Autodesk Inventor part; units mm, degrees
ref_plane "Work Plane1" through (227.2466, 0, 0) normal (0, 1, 0) x (-1, 0, 0)
ref_plane "YZ Plane" through (0, 0, 0) normal (1, 0, 0) x (0, 1, 0)
ref_plane "XZ Plane" through (0, 0, 0) normal (0, 1, 0) x (-1, 0, 0)
sketch "Sketch1" plane through (0, 0, 0) normal (0, 0, 1) x (1, 0, 0)
  line L0 (0, 0) -> (21, 0)
  line L1 (0, 0) -> (0, 80)
  line L2 (0, 80) -> (21, 80)
  line L3 (21, 80) -> (21, 0)
  line L4 (0, 96) -> (0, -16)
  line L5 (-4.2, 0) -> (25.2, 0)
  dimension "d1" = 160
  dimension "d2" = 21
revolve "Body" add sketch "Sketch1" angle 360 about axis through (0, 0, 0) along (1, 0, 0)
sketch "Sketch2" plane through (0, 0, 0) normal (-1, 0, 0) x (0, 0, 1)
  circle A0 centre (0, 0) radius 80
  point P0 (0, 0)
hole "Thread" at (0, 0, 0) direction (1, 0, 0) diameter 122.8349 end through all
chamfer "Chamfer1" distance 6 angle 30 1 edges at (0, -80, 0) measured on face at (0, -39.8141, -61.8966)
sketch "Sketch3" plane through (21, 0, 0) normal (1, 0, 0) x (0, 0, -1)
  circle A0 centre (0, 0) radius 80
  line L0 (-6, 79.7747) -> (-6, 75)
  line L1 (-6, 75) -> (6, 75)
  line L2 (6, 75) -> (6, 79.7747)
  line L3 (0, -112) -> (0, 112)
  line L4 (-112, 0) -> (112, 0)
  dimension "d12" = 6
  dimension "d13" = 6
  dimension "d14" = 75
extrude "Groove1" cut sketch "Sketch3" against normal through all contours L2 L1 L3 A0 | L3 L1 L0 A0
pattern_circular "Grooves1" count 4 over 360 about axis through (-10, 0, 0) along (1, 0, 0) of "Groove1"
fillet "Fillet1" radius 2.1 4 edges at (21, 56.5685, 56.5685) (21, 56.5685, -56.5685) (21, -56.5685, -56.5685) (21, -56.5685, 56.5685)
chamfer "Chamfer2" distance 3.125 angle 45 1 edges at (21, 0, -61.4175) measured on face at (21, -40.9181, 59.4692)
chamfer "Chamfer3" distance 3.125 angle 45 1 edges at (0, 0, -61.4175) measured on face at (0, 64.709, 25.6007)
ref_plane "Work Plane1" through (227.2466, 0, 0) normal (0, 1, 0) x (-1, 0, 0)
equation "\"d1\" = SD2"
equation "\"d2\" = KOH"
equation "\"d12\" = 0.5 * SNB"
equation "\"d13\" = 0.5 * SNB"
equation "\"d14\" = 0.5 * SD2 - SNT"
equation "\"d10\" = -0.5 * LADI + 0.5 * SD2"
equation "\"d11\" = FAWI2"
equation "\"d40\" = -0.5 * LADI + 0.5 * SD2"
equation "\"d18\" = RR"
equation "\"d19\" = 0.025 * NND"
equation "\"d41\" = 0.025 * NND"
equation "\"d21\" = 0.025 * NND"
equation "\"d42\" = 0.025 * NND"
equation "\"NND\" = 125"
equation "\"KOH\" = 21"
equation "\"SD2\" = 160"
equation "\"SNB\" = 12"
equation "\"SNT\" = 5"
equation "\"LADI\" = 148"
equation "\"RR\" = 2.1"
equation "\"FAWI2\" = 30deg"
equation "\"GUL\" = 0.61345 * PTC"
equation "\"THREADDIA\" = 125"
equation "\"TOA\" = 30deg"
equation "\"PTC\" = 2"
equation "\"GAL\" = 0.61345 * PTC"
equation "\"GD1\" = THREADDIA - 1.2269 * PTC"
properties part number "DIN 981 - KM 25" material "Steel, Mild"
Here's how the part is built. I have some questions about the finished solid (model axes, mm). A direction names the side the tool comes from. Give positions to 0.01 mm unless a question says otherwise; leave off trailing zeros. Order: outer loops, then holes, each group sorted by start corner. A loop starts at its lowest first (then second) coordinate and runs counter-clockwise, first axis right, second up. Notation, with made-up numbers: M -12.5,22.25 L -2.5,22.25 A15 ccw -2.5,46.25 Z; hole C 75,40.25 d3. An arc over 180 degrees is marked long. Use a Markdown table: item, result. Add a question column.
1. Suppose I cut it at B-B (x = 8.5). List the corners of the cut face in (y, z) for me, and give its area (3 significant figures).
2. For pin 1 Ø2 at (x, z) = (11.5, -60.5) entering from -Y; pin 2 Ø6 at (x, y) = (9.5, -36.5) entering from -Z; pin 3 Ø4 at (x, z) = (9, 76) entering from -Y, each with a flat end and sliding along its axis, tell me the tip position at first contact or that it passes through.
3. Suppose I cut it at A-A (y = 0). List the corners of the cut face in (x, z) for me (3 decimals).
4. I need wall thicknesses on probe 1 along Z at (x, y) = (9.75, 0); probe 2 along Y at (x, z) = (12.5, -17.5). Which ranges of each line are inside material? Lowest first, please. Write a range as from..to.
5. On a 3-axis mill with a long thin cutter (end or side, diameter ignored), from which of +Z, -Z, +X, -X, +Y, -Y can I reach the whole of each face in a straight line? I mean faces 1 (the flat face through (11, 77, -6)), 2 (the flat face through (11, 0, -75)), 3 (the flat face through (11, 0, 75)), 4 (the flat face through (11, -77, -6)). Say none if no direction works.
6. If we mould it in two halves opening along Z, with no side actions, what happens to faces 5 (the flat face through (11, 6, 77)), 6 (the flat face through (11, -77, 6)), 7 (the cylindrical face through (11.29, 57.13, 56))? For each: +Z half, -Z half, draft (parallel to the pull), parting line (faces both ways), or undercut.
Results list:
| question | item | result |
|---|---|---|
| 1 | outline | M -79.77,-6 A80 ccw -6,-79.77 L -6,-75 L 6,-75 L 6,-79.77 A80 ccw 79.77,-6 L 75,-6 L 75,6 L 79.77,6 A80 ccw 6,79.77 L 6,75 L -6,75 L -6,79.77 A80 ccw -79.77,6 L -75,6 L -75,-6 Z; hole C 0,0 d122.83 |
| 1 | area | 8,020 mm² |
| 2 | pin 1 | stops at y = -53.48 |
| 2 | pin 2 | stops at z = -72.65 |
| 2 | pin 3 | stops at y = -30.4 |
| 3 | outline | M 0,-74 L 0.577,-75 L 21,-75 L 21,-64.542 L 17.875,-61.417 L 3.125,-61.417 L 0,-64.542 Z; M 0,64.542 L 3.125,61.417 L 17.875,61.417 L 21,64.542 L 21,75 L 0.577,75 L 0,74 Z |
| 4 | probe 1 | z = -75..-61.42, 61.42..75 |
| 4 | probe 2 | y = -78.06..-58.87, 58.87..78.06 |
| 5 | face 1 | +X, -X, +Y |
| 5 | face 2 | -Z, +X, -X |
| 5 | face 3 | +Z, +X, -X |
| 5 | face 4 | +X, -X, -Y |
| 6 | face 5 | draft |
| 6 | face 6 | undercut |
| 6 | face 7 | +Z half |
